from build123d import *

# Parameters (mm, degrees)
SKETCH_W   = 95
SKETCH_H   = 70
SKETCH_R   = 8
SKETCH_R_2 = 11
PAD_DEPTH  = 10


with BuildPart() as part:
    # Sketch → Pad (new body)
    with BuildSketch(Plane.XY):
        with Locations((27.5, -15)):
            Rectangle(SKETCH_W, SKETCH_H)
        Circle(SKETCH_R, mode=Mode.SUBTRACT)
        with Locations((0, -30)):
            Circle(SKETCH_R_2, mode=Mode.SUBTRACT)
    extrude(amount=PAD_DEPTH)


solid = part.part
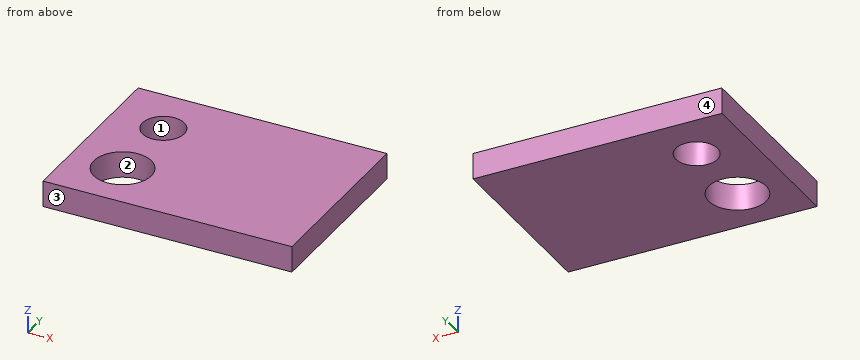
Input: part model. Units: mm. Frame: model coordinates. Face numbers are marked on the shaded views. Coordinates: 2 decimals unless noted, no trailing zeros. Loops run counter-clockwise (first coordinate to the right, second up) from the corner with the lowest first, then second, coordinate; pieces in that order, holes last. Notation, with made-up numbers: (60.5, -14) -> (96.5, -14) arc R6 ccw to (96.5, -3) -> close; hole circle Ø5 at (58.5, 24). An arc over 180 degrees is marked (long way). One line per item, written item: value.
(1) Cut plane D-D (y = -30). Output: boundary loops of the cut face in (x, z).
Answer below:
outline: (-20, 0) -> (-11, 0) -> (-11, 10) -> (-20, 10) -> close; (11, 0) -> (75, 0) -> (75, 10) -> (11, 10) -> close
(2) Cut plane B-B (x = 0). Output: boundary loops of the cut face in (y, z).
Answer below:
outline: (-50, 0) -> (-41, 0) -> (-41, 10) -> (-50, 10) -> close; (-19, 0) -> (-8, 0) -> (-8, 10) -> (-19, 10) -> close; (8, 0) -> (20, 0) -> (20, 10) -> (8, 10) -> close
(3) Cut plane C-C (z = 6). Output: boundary loops of the cut face in (x, y), then the cut area to 3 significant figures.
Answer below:
outline: (-20, -50) -> (75, -50) -> (75, 20) -> (-20, 20) -> close; hole circle Ø22 at (0, -30); hole circle Ø16 at (0, 0)
area: 6,070 mm2
(4) Draft query along Y for the marked faces 1, 2, 3 and 4. Return one class per face: pulls with the +Y half, pulls with the -Y half, needs draft (parallel to the pull), parting line crosses it, or undercut.
Answer below:
face 1: undercut
face 2: undercut
face 3: pulls with the -Y half
face 4: pulls with the +Y half
(5) Ray query, line 1 along Y through (x, z) = (0, 7.5); line 2 along X through (y, z) = (-25, 7.75); line 3 along Y through (x, z) = (9.5, 4.5). Return the intervals inside material, ascending.
Answer below:
line 1: y = -50 to -41, -19 to -8, 8 to 20
line 2: x = -20 to -9.8, 9.8 to 75
line 3: y = -50 to -35.55, -24.45 to 20
(6) Cut plane A-A (y = 0). Output: boundary loops of the cut face in (x, z).
Answer below:
outline: (-20, 0) -> (-8, 0) -> (-8, 10) -> (-20, 10) -> close; (8, 0) -> (75, 0) -> (75, 10) -> (8, 10) -> close
(7) Pin query (flat end, axial travel): pin 1 Ø9.5 at (x, y) = (0, 0) entering from -Z. Return the tip coordinate at first contact, or that it passes through.
Answer below:
pin 1: passes through
